from build123d import *

# Parameters (mm, degrees)
F0_R     = 17.5
F1_DEPTH = 25.4
F2_W     = 60.77839
F2_H     = 43.169699
F3_DEPTH = 25.4
F4_W     = 10
F4_H     = 25
F5_DEPTH = 40


with BuildPart() as f1:
    # F0 (on Top) → F1 (new body)
    with BuildSketch(Plane.XY):
        Circle(F0_R)
    extrude(amount=F1_DEPTH)

    # F2 (on Right) → F3 (cut)
    with BuildSketch(Plane.YZ):
        with Locations((0, 15.174311)):
            Rectangle(F2_W, F2_H)
    extrude(amount=-F3_DEPTH, mode=Mode.SUBTRACT)

    # F4 (on face) → F5 (cut)
    with BuildSketch(Plane.XY.offset(25.4)):
        with Locations((7, 0)):
            Rectangle(F4_W, F4_H)
    extrude(amount=-F5_DEPTH, mode=Mode.SUBTRACT)


solid = f1.part
Work out the finished part from the listing and answer in its coordinate system (mm). A direction names the side the tool comes from. Give positions to 0.01 mm unless a question says otherwise; leave off trailing zeros. Order: outer loops, then holes, each group sorted by start corner. A loop starts at its lowest first (then second) coordinate and runs counter-clockwise, first axis right, second up. Notation, with made-up numbers: (-29, 72.25) - (7, 72.25) arc R17 ccw to (7, 80.25) - close; hole circle Ø11 at (40, -28). An arc over 180 degrees is marked (long way). Answer as CSV lines item,"result". Start each with the question number.
Q1. The part is cut by section C-C (z = 23.75). Write down the section's boundary in (x, y), then the cut area to 3 significant figures.
Q2. The part is cut by section B-B (x = 6.25). Write down the section's boundary in (y, z), then the cut area to 3 significant figures.
Q3. Given pin 1 Ø1 at (x, z) = (13.5, 12) entering from -Y; pin 2 Ø8 at (x, z) = (9.5, 7) entering from -Y; pin 3 Ø3 at (y, z) = (-10, 20.5) entering from +X, each flat-ended and moving along its own axis, determine where each tip first touches the part or whether it passes through.
Q4. The part is cut by section D-D (x = 14.5). Write down the section's boundary in (y, z).
Q5. The mould has two halves that part along Y. Classify faces 1 (the face through (13, 0, 0)), 2 (the face through (7, 12.5, 13)), 3 (the face through (17.496, -0.385, 12.522)): +Y half, -Y half, draft (parallel to the pull), parting line (faces both ways), or undercut.
Q6. Find the intervals of material crossed by L1, parallel to X at y = -0.5, z = 7; L2, parallel to Y at x = 4.5, z = 17.5; L3, parallel to X at y = -5.5, z = 18.75, in increasing order. Write a range as [from, to].
Q7. The part is cut by section A-A (y = 0). Write down the section's boundary in (x, z).
Q8. For faces 4 (the face through (13, 0, 25.4)), 5 (the face through (7, -12.5, 13)), determine the directions among +Z, -Z, +X, -X, +Y, -Y from which every point of the face is accessible in a straight line to the end or side of a thin tool.
Check result:
1,outline,"(0, -17.5) arc R17.5 ccw to (0, 17.5) - close; hole (2, -12.5) - (12, -12.5) - (12, 12.5) - (2, 12.5) - close"
1,area,"231 mm²"
2,outline,"(-16.35, 0) - (-12.5, 0) - (-12.5, 25.4) - (-16.35, 25.4) - close; (12.5, 0) - (16.35, 0) - (16.35, 25.4) - (12.5, 25.4) - close"
2,area,"195 mm²"
3,pin 1,"stops at y = -11.72"
3,pin 2,"stops at y = -16.61"
3,pin 3,"stops at x = 15.3"
4,outline,"(-9.8, 0) - (9.8, 0) - (9.8, 25.4) - (-9.8, 25.4) - close"
5,face 1,"draft"
5,face 2,"undercut"
5,face 3,"parting line"
6,L1,"x = [0, 2], [12, 17.49]"
6,L2,"y = [-16.91, -12.5], [12.5, 16.91]"
6,L3,"x = [0, 2], [12, 16.61]"
7,outline,"(0, 0) - (2, 0) - (2, 25.4) - (0, 25.4) - close; (12, 0) - (17.5, 0) - (17.5, 25.4) - (12, 25.4) - close"
8,face 4,"+Z, +X, -X, +Y, -Y"
8,face 5,"+Z, -Z"
